Model file for the job. Use its own axes, mm. A direction names the side the tool comes from. Give positions to 0.01 mm unless a question says otherwise; leave off trailing zeros. Write each loop counter-clockwise with the first axis right and the second up, starting at its lowest first coordinate (ties: lowest second). Pieces come first, ordered by that corner, then holes.
```python
from build123d import *

# Parameters (mm, degrees)
CROQUIS1_R              = 7.25
SALIENTE_EXTRUIR1_DEPTH = 34
CROQUIS2_R              = 30.5
SALIENTE_EXTRUIR2_DEPTH = 24
CROQUIS3_R              = 7.25
CROQUIS2_2_R            = 30.5
REDONDEO1_R             = 5


# Read off the part's stored shape, not the designer's step: Vaciado1
with BuildPart() as part:
    # Croquis1 → Saliente-Extruir1 (new body)
    with BuildSketch(Plane(origin=(0, 0, 0), x_dir=(1, 0, 0), z_dir=(0, 1, 0))):
        with Locations(Location((0, 0, 0), (0, 0, 270))):
            Circle(CROQUIS1_R)
    extrude(amount=SALIENTE_EXTRUIR1_DEPTH)



with BuildPart() as body_2:
    # Croquis2 → Saliente-Extruir2 (new body)
    with BuildSketch(Plane(origin=(0, 47.8, 0), x_dir=(1, 0, 0), z_dir=(0, 1, 0))):
        with Locations(Location((0, 0, 0), (0, 0, 270))):
            Circle(CROQUIS2_R)
    extrude(amount=SALIENTE_EXTRUIR2_DEPTH)


with BuildPart() as part_1:
    add(part.part)

    add(body_2.part)  # Recubrir1 merges body 2
    # Croquis3 → Recubrir1 section 0
    with BuildSketch(Plane(origin=(0, 34, 0), x_dir=(1, 0, 0), z_dir=(0, 1, 0))):
        Circle(CROQUIS3_R)
    # Croquis2_2 → Recubrir1 section 1
    with BuildSketch(Plane(origin=(0, 47.8, 0), x_dir=(1, 0, 0), z_dir=(0, 1, 0))):
        Circle(CROQUIS2_2_R)
    loft()

    # Redondeo1
    redondeo1_edges = [part_1.edges().sort_by_distance(p)[0] for p in [
        (-21.566756826, 47.8, -21.566756826),
    ]]
    fillet(redondeo1_edges, radius=REDONDEO1_R)

    # Vaciado1 outline → Vaciado1 (revolve, cut)
    with BuildSketch(Plane.XY):
        with BuildLine():
            Line((29, 71.8), (0, 71.8))
            Line((0, 71.8), (0, 0))
            Line((0, 0), (5.75, 0))
            Line((5.75, 0), (5.75, 34.854003736))
            Line((5.75, 34.854003736), (27.286436978, 47.636921167))
            ThreePointArc((27.286436978, 47.636921167), (28.541589175, 48.91499344), (29, 50.646679119))
            Line((29, 50.646679119), (29, 71.8))
        make_face()
    revolve(axis=Axis((0, 0, 0), (0, 1, 0)), mode=Mode.SUBTRACT)


solid = part_1.part
```
1. Slice it at A-A, the plane y = 24.5. Write the cut outline in (x, z).
Calculated:
outline: circle Ø14.5 at (0, 0); hole circle Ø11.5 at (0, 0)
2. Slice it at B-B, the plane y = 64.5. Write the cut outline in (x, z), and give its area (3 significant figures).
Calculated:
outline: circle Ø61 at (0, 0); hole circle Ø58 at (0, 0)
area: 280 mm2
3. Pull direction Z, two halves, no side cores. Call faces 1 (the cylindrical face through (-2.777, 16.762, 6.697)), 2 (the flat face through (-11, 71.8, 27)), 3 (the cylindrical face through (-0.75, 17.67, -5.7)): +Z half, -Z half, draft (parallel to the pull), parting line (faces both ways), or undercut.
Calculated:
face 1: parting line
face 2: draft
face 3: undercut
4. Which spindle directions (+Z, -Z, +X, -X, +Y, -Y) get a long thin tool onto all of the face, cutting with end or side? Do faces 4 (the cylindrical face through (-27.06, 61.07, 14.07)), 5 (the cylindrical face through (13.38, 61.37, 25.73)). Say none if no direction does.
Calculated:
face 4: +Y, -Y
face 5: +Y
5. Pin check, flat tips, straight feed: P1, Ø3, axis at y = 9, z = -3.5, coming from the +X side; P2, Ø1.5, axis at x = -14, z = 19, coming from the +Y side; P3, Ø8, axis at x = 18.5, y = 56, coming from the -Z side. Stop position of each tip, or through.
Calculated:
P1: stops at x = 6.97
P2: stops at y = 45.89
P3: stops at z = -26.83
6. Probe probe 1 along X at (y, z) = (19, 0); probe 2 along X at (y, z) = (61, 0). List the from-to ranges inside material, lowest first.
Calculated:
probe 1: x = -7.25 to -5.75, 5.75 to 7.25
probe 2: x = -30.5 to -29, 29 to 30.5
